Autodesk Fusion 360 part; units mm, degrees
sketch "Sketch1" plane through (0, 0, 0) normal (0, 0, 1) x (1, 0, 0)
  circle A0 centre (0, 0) radius 3
  line L0 (0, 0) -> (35, 0)
  line L1 (35, 0) -> (35, 3)
  line L2 (14, 4) -> (11, 4)
  line L3 (0, 3) -> (0, 0)
  line L4 (0, 0) -> (35, 0)
  line L5 (35, 0) -> (35, -3)
  line L6 (14, -4) -> (11, -4)
  line L7 (0, -3) -> (0, 0)
  line L8 (35, 0) -> (21, 0)
  line L9 (21, 0) -> (21, 2)
  line L10 (21, 2) -> (35, 2)
  line L11 (35, 2) -> (35, 0)
  line L12 (35, 0) -> (21, 0)
  line L13 (21, 0) -> (21, -2)
  line L14 (21, -2) -> (35, -2)
  line L15 (35, -2) -> (35, 0)
  line L16 (35, 2) -> (35, 3)
  line L17 (35, -2) -> (35, -3)
  line L18 (0, 0) -> (12.5, 0)
  line L19 (12.5, 0) -> (12.5, 1.5)
  line L20 (12.5, 0) -> (12.5, -1.5)
  circle A1 centre (12.5, 1.5) radius 0.5
  circle A2 centre (12.5, -1.5) radius 0.5
  line L21 (0, 3) -> (11, 4)
  line L22 (35, 3) -> (14, 4)
  line L23 (0, -3) -> (11, -4)
  line L24 (35, -3) -> (14, -4)
  dimension "d1" = 6
  dimension "d2" = 35
  dimension "d3" = 14
  dimension "d4" = 14
  dimension "d5" = 12.5
  dimension "d6" = 1.5
  dimension "d7" = 1.5
  dimension "d8" = 1
  dimension "d9" = 1
extrude "Extrude1" add sketch "Sketch1" along normal blind 4 makes body 1
sketch "Sketch2" plane through (0, 0, 0) normal (0, 0, -1) x (1, 0, 0)
  circle A0 centre (12.5, -1.5) radius 0.5
  circle A1 centre (12.5, 1.5) radius 0.5
  line L0 (35, -3) -> (35, 2)
  line L1 (35, 2) -> (35, 3)
  line L2 (35, 3) -> (14, 4)
  line L3 (14, 4) -> (11, 4)
  line L4 (11, 4) -> (0, 3)
  arc A2 (0, 3) -> (0, -3) centre (0, 0) ccw
  line L5 (0, -3) -> (11, -4)
  line L6 (11, -4) -> (14, -4)
  line L7 (14, -4) -> (35, -3)
  line L8 (35, 3) -> (35, -3)
  line L9 (35, 0) -> (21, 0)
  line L10 (21, 0) -> (21, 2)
  line L11 (21, 2) -> (35, 2)
  line L12 (35, 2) -> (35, 0)
  line L13 (35, 0) -> (21, 0)
  line L14 (21, 0) -> (21, -2)
  line L15 (21, -2) -> (35, -2)
  line L16 (35, -2) -> (35, 0)
  dimension "d12" = 14
  dimension "d13" = 2
extrude "Extrude2" cut sketch "Sketch2" against normal blind 3 contours L0 L8 L9 L13 L14 L15 L16 | L0 L8 L9 L10 L11 L12 L13 bodies 1
sketch "Sketch3" plane through (0, 0, 4) normal (0, 0, 1) x (-1, 0, 0)
  circle A0 centre (-12.5, -1.5) radius 0.5
  circle A1 centre (-12.5, 1.5) radius 0.5
  line L0 (-35, 2) -> (-35, -3)
  line L1 (-35, -3) -> (-14, -4)
  line L2 (-14, -4) -> (-11, -4)
  line L3 (-11, -4) -> (0, -3)
  arc A2 (0, -3) -> (0, 3) centre (0, 0) ccw
  line L4 (0, 3) -> (-11, 4)
  line L5 (-11, 4) -> (-14, 4)
  line L6 (-14, 4) -> (-35, 3)
  line L7 (-35, 3) -> (-35, 2)
  circle A3 centre (0, 0) radius 3
  dimension "d16" = 6
extrude "Extrude3" cut sketch "Sketch3" against normal blind 1 contours A2 A3 bodies 1
sketch "Sketch4" plane through (0, 0, 0) normal (0, 0, -1) x (1, 0, 0)
  line L0 (21, 2) -> (35, 2)
  line L1 (35, 2) -> (35, 3)
  line L2 (35, 3) -> (14, 4)
  line L3 (14, 4) -> (11, 4)
  line L4 (11, 4) -> (0, 3)
  arc A0 (0, 3) -> (0, -3) centre (0, 0) ccw
  line L5 (0, -3) -> (11, -4)
  line L6 (11, -4) -> (14, -4)
  line L7 (14, -4) -> (35, -3)
  line L8 (35, -3) -> (35, -2)
  line L9 (35, -2) -> (21, -2)
  line L10 (21, -2) -> (21, 2)
  circle A1 centre (12.5, -1.5) radius 0.5
  circle A2 centre (12.5, 1.5) radius 0.5
  circle A3 centre (0, 0) radius 3
  dimension "d19" = 6
extrude "Extrude4" cut sketch "Sketch4" against normal blind 1 contours A0 A3 bodies 1
sketch "Sketch5" plane through (0, 0, 4) normal (0, 0, 1) x (-1, 0, 0)
  arc A0 (0, 3) -> (0, -3) centre (0, 0) ccw
  line L0 (0, 3) -> (-11, 4)
  line L1 (-11, 4) -> (-14, 4)
  line L2 (-14, 4) -> (-35, 3)
  line L3 (-35, 3) -> (-35, 2)
  line L4 (-35, 2) -> (-35, -3)
  line L5 (-35, -3) -> (-14, -4)
  line L6 (-14, -4) -> (-11, -4)
  line L7 (-11, -4) -> (0, -3)
  circle A1 centre (-12.5, -1.5) radius 0.5
  circle A2 centre (-12.5, 1.5) radius 0.5
  line L8 (-3, 0) -> (-0.0018, 0)
  line L9 (-0.0018, 0) -> (-0.0018, -3.5)
  line L10 (-0.0018, -3.5) -> (-3, -3.5)
  line L11 (-3, -3.5) -> (-3, 0)
extrude "Extrude5" cut sketch "Sketch5" against normal blind 1 contours A0 L7 L11 bodies 1
sketch "Sketch6" plane through (0, 0, 4) normal (0, 0, 1) x (-1, 0, 0)
  circle A0 centre (-12.5, 1.5) radius 0.5
  circle A1 centre (-12.5, -1.5) radius 0.5
  line L0 (-3, -3.2727) -> (-3, 0)
  arc A2 (0, 3) -> (-3, 0) centre (0, 0) ccw
  line L1 (0, 3) -> (-11, 4)
  line L2 (-11, 4) -> (-14, 4)
  line L3 (-14, 4) -> (-35, 3)
  line L4 (-35, 3) -> (-35, 2)
  line L5 (-35, 2) -> (-35, -3)
  line L6 (-35, -3) -> (-14, -4)
  line L7 (-14, -4) -> (-11, -4)
  line L8 (-11, -4) -> (-3, -3.2727)
  line L9 (-3, 0) -> (0.4438, 0)
  line L10 (0.4438, 0) -> (0.4438, 3.5)
  line L11 (0.4438, 3.5) -> (-3, 3.5)
  line L12 (-3, 3.5) -> (-3, 0)
extrude "Extrude6" cut sketch "Sketch6" against normal blind 1 contours A2 L1 L12 bodies 1
sketch "Sketch7" plane through (0, 0, 0) normal (0, 0, -1) x (1, 0, 0)
  circle A0 centre (12.5, 1.5) radius 0.5
  circle A1 centre (12.5, -1.5) radius 0.5
  arc A2 (0, -3) -> (0, 3) centre (0, 0) ccw
  line L0 (0, -3) -> (11, -4)
  line L1 (11, -4) -> (14, -4)
  line L2 (14, -4) -> (35, -3)
  line L3 (35, -3) -> (35, -2)
  line L4 (35, -2) -> (21, -2)
  line L5 (21, -2) -> (21, 2)
  line L6 (21, 2) -> (35, 2)
  line L7 (35, 2) -> (35, 3)
  line L8 (35, 3) -> (14, 4)
  line L9 (14, 4) -> (11, 4)
  line L10 (11, 4) -> (0, 3)
  line L11 (3, 0) -> (0, 0)
  line L12 (0, 0) -> (0, 3.3794)
  line L13 (0, 3.3794) -> (3, 3.3794)
  line L14 (3, 3.3794) -> (3, 0)
extrude "Extrude7" cut sketch "Sketch7" against normal blind 1 contours A2 L10 L14 bodies 1
sketch "Sketch8" plane through (0, 0, 0) normal (0, 0, -1) x (1, 0, 0)
  line L0 (3, 3.2727) -> (3, 0)
  arc A0 (0, -3) -> (3, 0) centre (0, 0) ccw
  line L1 (0, -3) -> (11, -4)
  line L2 (11, -4) -> (14, -4)
  line L3 (14, -4) -> (35, -3)
  line L4 (35, -3) -> (35, -2)
  line L5 (35, -2) -> (21, -2)
  line L6 (21, -2) -> (21, 2)
  line L7 (21, 2) -> (35, 2)
  line L8 (35, 2) -> (35, 3)
  line L9 (35, 3) -> (14, 4)
  line L10 (14, 4) -> (11, 4)
  line L11 (11, 4) -> (3, 3.2727)
  circle A1 centre (12.5, -1.5) radius 0.5
  circle A2 centre (12.5, 1.5) radius 0.5
  line L12 (3, 0) -> (-0.0333, 0)
  line L13 (-0.0333, 0) -> (-0.0333, -3.5)
  line L14 (-0.0333, -3.5) -> (3, -3.5)
  line L15 (3, -3.5) -> (3, 0)
extrude "Extrude8" cut sketch "Sketch8" against normal blind 1 contours A0 L1 L15 bodies 1
sketch "Sketch9" plane through (0, 0, 3) normal (0, 0, 1) x (-1, 0, 0)
  arc A0 (0, -3) -> (0, 3) centre (0, 0) ccw
  line L0 (0, 3) -> (-3, 3.2727)
  line L1 (-3, 3.2727) -> (-3, -3.2727)
  line L2 (-3, -3.2727) -> (-0.0018, -3.0002)
  line L3 (-0.0018, -3.0002) -> (-0.0018, -3)
  arc A1 (-0.0018, -3) -> (0, -3) centre (0, 0) ccw
  circle A2 centre (0, 0) radius 0.5
  dimension "d30" = 1
hole "Hole1" at (0, 0, 3) direction (0, 0, -1) diameter 1 depth 2 tip angle 180 bodies 1
fillet "Fillet1" radius 0.5 10 edges at (35, -2.5, 4) (35, 0.5, 4) (35, 3, 2) (24.5, 3.5, 4) (35, -3, 2) (24.5, -3.5, 4) (12.5, -4, 4) (7, -3.6364, 4) (7, 3.6364, 4) (12.5, 4, 4) on bodies 1
extrude "Extrude9" cut 1 faces at (3, -0.9236, 3.3333) along direction (-1, 0, 0) blind 6.8 on bodies 1 bodies 1 makes body 2
delete_body "RemoveBody1" bodies 2
Geometry check sheet. Reference: the model listing, model coordinates, mm. A direction names the side the tool comes from. Round coordinates to 2 decimals unless told otherwise and drop trailing zeros. Loops run counter-clockwise (first coordinate to the right, second up) from the corner with the lowest first, then second, coordinate; pieces in that order, holes last. Notation, with made-up numbers: (87, 7.25) - (91, 7.25) arc R28 ccw to (91, 40.25) - close; hole circle Ø11 at (77, -36). An arc over 180 degrees is marked (long way). Write each question's results on one line, items separated by ' | '. Start each with the question number.
Q1. Cross-section at D-D on z = 0.5. Enter the section's corners in (x, y), and give its area (3 significant figures).
Q2. Thickness scan on line 1 (Y direction, x = 12.5, z = 2.35); line 2 (Y direction, x = 0, z = 2.1); line 3 (X direction, y = -1.75, z = 2.6). Record the ranges inside material, lowest first. Write a range as [from, to].
Q3. Release check for a two-part mould opening along Y. For faces 1 (the cylindrical face through (6.934, -3.487, 3.85)), 2 (the flat face through (6.6, 3.6, 1.7)), 3 (the cylindrical face through (12.962, 1.692, 1.972)) record: +Y half, -Y half, draft (parallel to the pull), parting line (faces both ways), or undercut.
Q4. Cross-section at B-B on y = 0. Enter the section's corners in (x, z).
Q5. Access from +Z, -Z, +X, -X, +Y, -Y to the whole of each face (thin tool, end or side, straight path). Record for faces 4 (the flat face through (1, 0, 1)), 5 (the flat face through (28, 2, 1)), 6 (the flat face through (3, 0, 3.5)).
Q6. Cross-section at C-C on z = 2.1. Enter the section's corners in (x, y), and give its area (3 significant figures).
Q7. Cross-section at A-A on x = 12.5. Enter the section's corners in (y, z).
Q8. Gauge pin test, flat ends, axial feed: P1, Ø1, axis at x = 24.5, z = 1.5, coming from the -Y side; P2, Ø1.2, axis at x = 29, y = 0.5, coming from the -Z side; P3, Ø3, axis at x = 1, y = -1, coming from the -Z side; P4, Ø1, axis at x = 18, y = -1, coming from the -Z side. Record the tip position at first contact, or that the pin passes through.
Answers below:
1) outline: (3, -3.27) - (11, -4) - (14, -4) - (34.52, -3.02) arc R0.5 ccw to (35, -2.52) - (35, -2) - (21, -2) - (21, 2) - (35, 2) - (35, 2.52) arc R0.5 ccw to (34.52, 3.02) - (14, 4) - (11, 4) - (3, 3.27) - close; hole circle Ø1 at (12.5, -1.5); hole circle Ø1 at (12.5, 1.5) | area: 172 mm²
2) line 1: y = [-4, -2], [-1, 1], [2, 4] | line 2: y = [-3, -0.5], [0.5, 3] | line 3: x = [-2.44, 12.07], [12.93, 21]
3) face 1: -Y half | face 2: +Y half | face 3: undercut
4) outline: (-3, 1) - (-0.5, 1) - (-0.5, 3) - (-3, 3) - close; (0.5, 1) - (3, 1) - (3, 0) - (21, 0) - (21, 3) - (35, 3) - (35, 3.5) arc R0.5 ccw to (34.5, 4) - (3, 4) - (3, 3) - (0.5, 3) - close
5) face 4: -Z, -X, +Y, -Y | face 5: -Z, +X | face 6: +Z, -X, +Y, -Y
6) outline: (0, -3) - (11, -4) - (14, -4) - (34.52, -3.02) arc R0.5 ccw to (35, -2.52) - (35, -2) - (21, -2) - (21, 2) - (35, 2) - (35, 2.52) arc R0.5 ccw to (34.52, 3.02) - (14, 4) - (11, 4) - (0, 3) arc R3 ccw to start; hole circle Ø1 at (0, 0); hole circle Ø1 at (12.5, -1.5); hole circle Ø1 at (12.5, 1.5) | area: 204 mm²
7) outline: (-4, 0) - (-2, 0) - (-2, 4) - (-3.5, 4) arc R0.5 ccw to (-4, 3.5) - close; (-1, 0) - (1, 0) - (1, 4) - (-1, 4) - close; (2, 0) - (4, 0) - (4, 3.5) arc R0.5 ccw to (3.5, 4) - (2, 4) - close
8) P1: stops at y = -3.52 | P2: stops at z = 3 | P3: stops at z = 1 | P4: stops at z = 0
